Input: part model. Units: mm. Frame: model coordinates. Coordinates: 2 decimals unless noted, no trailing zeros. Write each loop counter-clockwise with the first axis right and the second up, starting at its lowest first coordinate (ties: lowest second). Pieces come first, ordered by that corner, then holes. Notation, with made-up numbers: M 25,25.25 L 60,25.25 A23 cw 60,48.25 Z; hole C -39.5,39 d1. An arc over 180 degrees is marked long. Use one line per item in the form item = value.
from build123d import *

# Parameters (mm, degrees)
F0_W     = 40
F0_H     = 40
F1_DEPTH = 6
F2_R     = 15
F3_R     = 1.5
F4_DEPTH = 2


with BuildPart() as f1:
    # F0 (on Top) → F1 (new body)
    with BuildSketch(Plane.XY):
        Rectangle(F0_W, F0_H)
    extrude(amount=F1_DEPTH)

    # F2
    f2_edges = [f1.edges().sort_by_distance(p)[0] for p in [
        (-20, 20, 3),
        (20, 20, 3),
        (20, -20, 3),
        (-20, -20, 3),
    ]]
    fillet(f2_edges, radius=F2_R)

    # F3 (on face) → F4 (cut)
    with BuildSketch(Plane(origin=(0, 0, 0), x_dir=(1, 0, 0), z_dir=(0, 0, -1))):
        Circle(F3_R)
    extrude(amount=-F4_DEPTH, mode=Mode.SUBTRACT)

    # F5 (on Front) → F6 (revolve, cut)
    with BuildSketch(Plane.XZ):
        Polygon((0, 0), (0, 2), (-15, 0), align=None)
    revolve(axis=Axis((0, 0, 1), (0, 0, -1)), mode=Mode.SUBTRACT)


solid = f1.part
(1) Section query D-D on y = 17. Return the cut outline in (x, z), plus the area to 3 significant figures.
Computed:
outline = M -14,0 L 14,0 L 14,6 L -14,6 Z
area = 168 mm^2
(2) Pull-direction query (X, two-part tool) for faces 1 (the flat face through (0, 0, 6)), 2 (the cylindrical face through (-15.72, 15.49, 3.04)), 3 (the flat face through (0, 0, 2)); classes: pulls with the +X half, pulls with the -X half, needs draft (parallel to the pull), parting line crosses it, or undercut.
Computed:
face_1 = needs draft
face_2 = pulls with the -X half
face_3 = undercut
(3) Section query C-C on z = 5. Return the cut outline in (x, y), plus the area to 3 significant figures.
Computed:
outline = M -20,-5 A15 ccw -5,-20 L 5,-20 A15 ccw 20,-5 L 20,5 A15 ccw 5,20 L -5,20 A15 ccw -20,5 Z
area = 1,410 mm^2
(4) First-contact query: pin 1 Ø2 at (x, z) = (12, 3) entering from -Y; pin 2 Ø1.5 at (x, y) = (0.5, -0.5) entering from -Z; pin 3 Ø1.5 at (x, z) = (-12.5, 4.5) entering from +Y. Flat tips, straight axial feed; report the tip coordinate or a pass-through.
Computed:
pin_1 = -18.75
pin_2 = 2
pin_3 = 18.4
(5) Section query A-A on x = 0. Return the cut outline in (y, z).
Computed:
outline = M -20,0 L -15,0 L -1.5,1.8 L -1.5,2 L 1.5,2 L 1.5,1.8 L 15,0 L 20,0 L 20,6 L -20,6 Z
(6) Line query: probe 1 along X at (y, z) = (0, 1.95); probe 2 along Z at (x, y) = (-8.5, -8.5). Output: solid intervals per line, ascending.
Computed:
probe_1 = -20 to -1.5, 1.5 to 20
probe_2 = 0.4 to 6
